Job drawing, mm, ordinate dimensions from the low corner. One solid piece. Give positions to 0.01 mm unless a question says otherwise; leave off trailing zeros. Loops run counter-clockwise (first coordinate to the right, second up) from the corner with the lowest first, then second, coordinate; pieces in that order, holes last. Notation, with made-up numbers: M 87.25,60.5 L 119.25,60.5 A25 cw 119.25,76.5 Z; hole C 41,52.5 d1. An arc over 180 degrees is marked long. Answer in a Markdown table with one row per item.
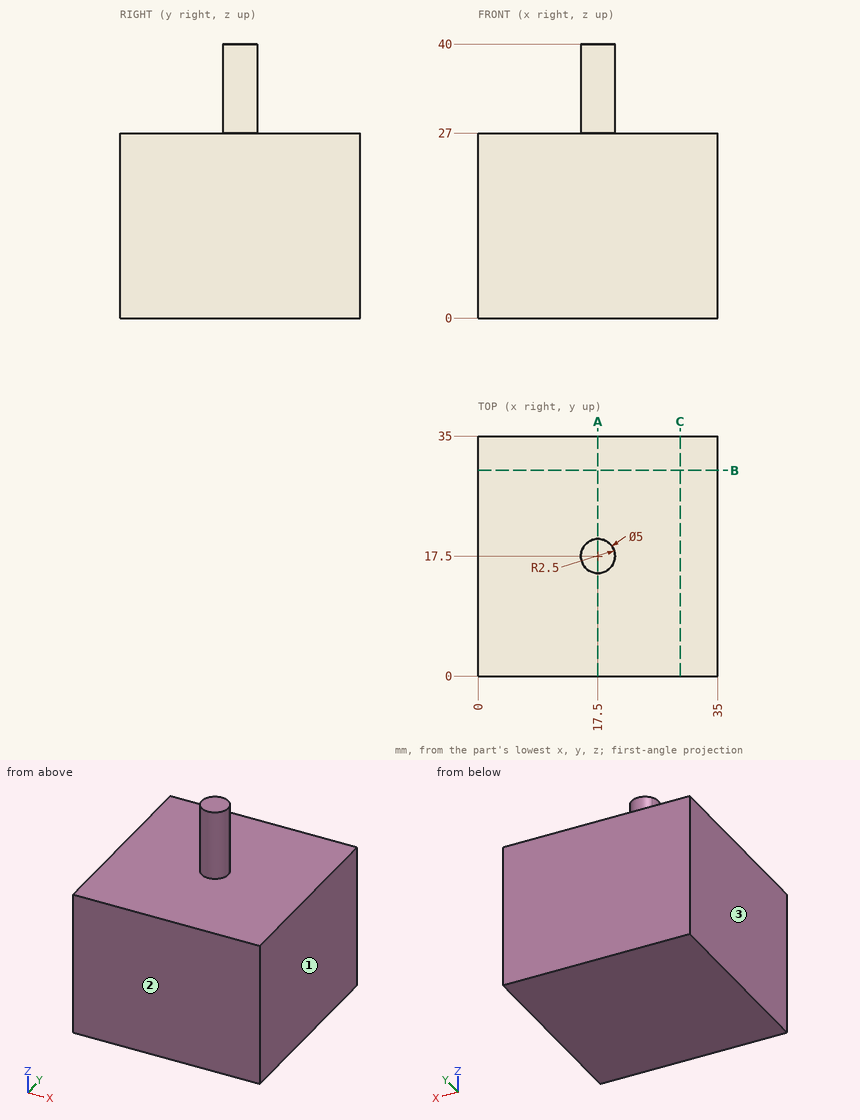
(1) Pull direction X, two halves, no side cores. Call the marked faces 1, 2 and 3: +X half, -X half, draft (parallel to the pull), parting line (faces both ways), or undercut.
Recorded:
| item | result |
|---|---|
| face 1 | +X half |
| face 2 | draft |
| face 3 | -X half |
(2) Drill centre lines: line 1 along Z through (x, y) = (30.5, 11); line 2 along Y through (x, z) = (18.5, 30). Where is each one in solid material? Low to high.
Recorded:
| item | result |
|---|---|
| line 1 | z = 0 to 27 |
| line 2 | y = 15.21 to 19.79 |
(3) Pin check, flat tips, straight feed: pin 1 Ø5 at (y, z) = (17.5, 30.5) entering from -X; pin 2 Ø1 at (x, y) = (17, 25.5) entering from +Z. Stop position of each tip, or through.
Recorded:
| item | result |
|---|---|
| pin 1 | stops at x = 15 |
| pin 2 | stops at z = 27 |
(4) Saw through at B-B (y = 30). Write the cut outline in (x, z), plus the area to 3 significant figures.
Recorded:
| item | result |
|---|---|
| outline | M 0,0 L 35,0 L 35,27 L 0,27 Z |
| area | 945 mm^2 |
(5) Saw through at A-A (x = 17.5). Write the cut outline in (y, z).
Recorded:
| item | result |
|---|---|
| outline | M 0,0 L 35,0 L 35,27 L 20,27 L 20,40 L 15,40 L 15,27 L 0,27 Z |
